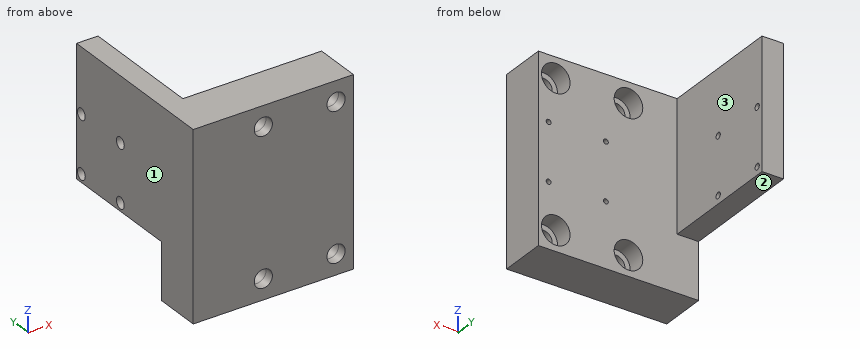
Autodesk Inventor part; units mm, degrees
ref_plane "YZ Plane" through (0, 0, 0) normal (1, 0, 0) x (0, 1, 0)
ref_plane "XZ Plane" through (0, 0, 0) normal (0, 1, 0) x (-1, 0, 0)
ref_plane "XY Plane" through (0, 0, 0) normal (0, 0, 1) x (1, 0, 0)
sketch "Sketch1" plane through (0, 0, 0) normal (0, 0, 1) x (1, 0, 0)
  line L0 (0, 0) -> (7.5, 0)
  line L1 (7.5, 13) -> (7.5, 56.5)
  line L2 (7.5, 56.5) -> (0, 56.5)
  line L3 (0, 56.5) -> (0, 0)
  line L4 (0, 0) -> (56, 0)
  line L5 (56, 0) -> (56, 13)
  line L6 (56, 13) -> (7.5, 13)
  line L7 (0, 13) -> (0, 0)
  dimension "d0" = 13
  dimension "d1" = 56
  dimension "d2" = 56.5
  dimension "d3" = 7.5
extrude "Extrusion1" add sketch "Sketch1" along normal mid plane 65
sketch "Sketch2" plane through (7.5, 13, 32.5) normal (0, 1, 0) x (1, 0, 0)
  line L0 (0, 0) -> (48.5, 0)
  line L1 (48.5, 0) -> (48.5, 65)
  line L2 (48.5, 65) -> (0, 65)
  line L3 (0, 0) -> (0, 65)
  line L4 (42.414, 25.5) -> (42.414, 39.5)
  line L5 (49.414, 32.5) -> (35.414, 32.5)
  point P0 (-7.5, 32.5)
  point P1 (17.014, 57.9)
  point P2 (17.014, 7.1)
  point P3 (42.414, 57.9)
  point P4 (42.414, 7.1)
  dimension "d6" = 25.4
  dimension "d7" = 25.4
  dimension "d8" = 25.4
  dimension "d9" = 25.4
  dimension "d10" = 25.4
  dimension "d11" = 25.4
  dimension "d35" = 25.4
hole "Hole1" at (24.514, 13, -25.4) at (24.514, 13, 25.4) at (49.914, 13, -25.4) at (49.914, 13, 25.4) direction (0, -1, 0) diameter 6.35 end through all counterbore diameter 10 counterbore depth 6.5
sketch "Sketch3" plane through (7.5, 13, 32.5) normal (0, 1, 0) x (1, 0, 0)
  circle A0 centre (24.9141, 42.5) radius 2.032
  circle A1 centre (24.9141, 22.5) radius 2.032
  circle A2 centre (44.914, 22.5) radius 1.143
  circle A3 centre (44.914, 42.5) radius 1.143
  point P0 (-7.5, 32.5)
hole "Hole2" at (52.414, 13, -10) at (52.414, 13, 10) at (32.4141, 13, 10) at (32.4141, 13, -10) direction (0, -1, 0) diameter 1.694 depth 4 tip angle 118
sketch "Sketch4" plane through (0, 0, 32.5) normal (-1, 0, 0) x (0, 0, 1)
  line L0 (0, 56.5) -> (0, 13)
  line L1 (0, 13) -> (-65, 13)
  line L2 (-65, 13) -> (-65, 56.5)
  line L3 (0, 56.5) -> (-65, 56.5)
  circle A0 centre (-42.5044, 54.0403) radius 0.889
  circle A1 centre (-22.5044, 34.0403) radius 0.889
  circle A2 centre (-22.5044, 54.0403) radius 1.0922
  line L4 (-45.0044, 32.0483) -> (-45.0044, 31.5403)
  line L5 (-45.0044, 31.5403) -> (-20.0044, 31.5403)
  line L6 (-20.0044, 31.5403) -> (-20.0044, 56.5403)
  line L7 (-20.0044, 56.5403) -> (-45.0044, 56.5403)
  line L8 (-45.0044, 56.5403) -> (-45.0044, 56.0323)
  line L9 (-45.0044, 56.0323) -> (-45.3092, 56.0323)
  line L10 (-45.3092, 32.0483) -> (-45.3092, 56.0323)
  line L11 (-45.0044, 32.0483) -> (-45.3092, 32.0483)
  circle A3 centre (-42.5044, 34.0403) radius 0.889
  circle A4 centre (-22.5044, 34.0403) radius 0.889
  circle A5 centre (-42.5044, 54.0403) radius 0.889
  circle A6 centre (-22.5044, 54.0403) radius 0.889
  circle A7 centre (-38.8544, 37.6903) radius 1.7272
  circle A8 centre (-26.1544, 37.6903) radius 1.7272
  circle A9 centre (-38.8544, 50.3903) radius 1.7272
  circle A10 centre (-26.1544, 50.3903) radius 1.7272
  circle A11 centre (-32.5044, 44.0403) radius 1.7272
  point P0 (-32.5, 0)
hole "Hole3" at (0, 54.0403, -10.0044) at (0, 54.0403, 9.9956) at (0, 34.0403, 9.9956) at (0, 34.0403, -10.0044) direction (1, 0, 0) diameter 2.1844 end through all counterbore diameter 4 counterbore depth 3
sketch "Sketch5" plane through (7.5, 13, 32.5) normal (1, 0, 0) x (0, 0, -1)
  line L0 (0, 0) -> (65, 0)
  line L1 (45.3092, 19.0483) -> (45.3092, 43.0323)
  line L2 (65, 43.5) -> (45.3092, 43.5)
  line L3 (45.3092, 43.5) -> (45.3092, 0)
  line L4 (45.3092, 0) -> (65, 0)
  line L5 (65, 0) -> (65, 43.5)
  point P0 (32.5, -13)
extrude "Extrusion2" cut sketch "Sketch5" against normal blind 10
sketch "Sketch6" plane through (0, 0, 32.5) normal (0, -1, 0) x (1, 0, 0)
  circle A0 centre (49.914, -7.1) radius 3.175
  circle A1 centre (49.914, -57.9) radius 3.175
  circle A2 centre (24.514, -7.1) radius 3.175
  circle A3 centre (24.514, -57.9) radius 3.175
  line L0 (56, 0) -> (0, 0)
  line L1 (0, -65) -> (0, 0)
  line L2 (0, -65) -> (56, -65)
  line L3 (56, 0) -> (56, -65)
  point P0 (0, -32.5)
extrude "Extrusion3" add sketch "Sketch6" along normal blind 3.3198
properties part number "beam steering subassy mounting bracket"
Part model, mm, in its own coordinate system. Face numbers are marked on the shaded views. A direction names the side the tool comes from. Give positions to 0.01 mm unless a question says otherwise; leave off trailing zeros. Order: outer loops, then holes, each group sorted by start corner. A loop starts at its lowest first (then second) coordinate and runs counter-clockwise, first axis right, second up. Notation, with made-up numbers: (33, 69.25) -> (43, 69.25) arc R29 cw to (43, 108.25) -> close; hole circle Ø10 at (86.5, 80.25). An arc over 180 degrees is marked (long way). Use one line per item in the form item = value.
(1) Saw through at C-C (x = 12). Write the cut outline in (y, z).
Solution:
outline = (-3.32, -32.5) -> (13, -32.5) -> (13, 32.5) -> (-3.32, 32.5) -> close
(2) Saw through at B-B (z = -25.4). Write the cut outline in (x, y).
Solution:
outline = (0, -3.32) -> (21.34, -3.32) -> (21.34, 6.5) -> (19.51, 6.5) -> (19.51, 13) -> (0, 13) -> close; (27.69, -3.32) -> (46.74, -3.32) -> (46.74, 6.5) -> (44.91, 6.5) -> (44.91, 13) -> (29.51, 13) -> (29.51, 6.5) -> (27.69, 6.5) -> close; (53.09, -3.32) -> (56, -3.32) -> (56, 13) -> (54.91, 13) -> (54.91, 6.5) -> (53.09, 6.5) -> close
(3) Saw through at D-D (y = 22.5). Write the cut outline in (x, z).
Solution:
outline = (0, -12.81) -> (7.5, -12.81) -> (7.5, 32.5) -> (0, 32.5) -> close
(4) Flat gauge pins, fed straight in: P1, Ø4, axis at y = 36.5, z = 21.5, coming from the +X side; P2, Ø8, axis at x = 3, y = 29.5, coming from the -Z side; P3, Ø16, axis at x = 49.914, z = 25.4, coming from the +Y side. Where does each tip first touch, or does it go through?
Solution:
P1 = 7.5
P2 = -12.81
P3 = 13
(5) Saw through at A-A (z = 25.4). Write the cut outline in (x, y), then the cut area to 3 significant figures.
Solution:
outline = (0, -3.32) -> (21.34, -3.32) -> (21.34, 6.5) -> (19.51, 6.5) -> (19.51, 13) -> (7.5, 13) -> (7.5, 56.5) -> (0, 56.5) -> close; (27.69, -3.32) -> (46.74, -3.32) -> (46.74, 6.5) -> (44.91, 6.5) -> (44.91, 13) -> (29.51, 13) -> (29.51, 6.5) -> (27.69, 6.5) -> close; (53.09, -3.32) -> (56, -3.32) -> (56, 13) -> (54.91, 13) -> (54.91, 6.5) -> (53.09, 6.5) -> close
area = 985 mm²
(6) Drill centre lines: line 1 (X direction, y = 11, z = -25); line 2 (X direction, y = 11.9, z = -10); line 3 (X direction, y = 26.5, z = 27.5). Where is each one in solid material? Low to high. Write a range as from..to.
Solution:
line_1 = 0..19.53, 29.5..44.93, 54.9..56
line_2 = 0..31.57, 33.26..51.57, 53.26..56
line_3 = 0..7.5
(7) Tool access for the marked faces 1, 2 and 3: list every direction of +Z, -Z, +X, -X, +Y, -Y with a clear straight run to the whole face (end or side of a thin tool).
Solution:
face_1 = +Z, -Z, -X, +Y, -Y
face_2 = -Z, +X, -X, +Y
face_3 = +Z, -Z, +X, +Y
